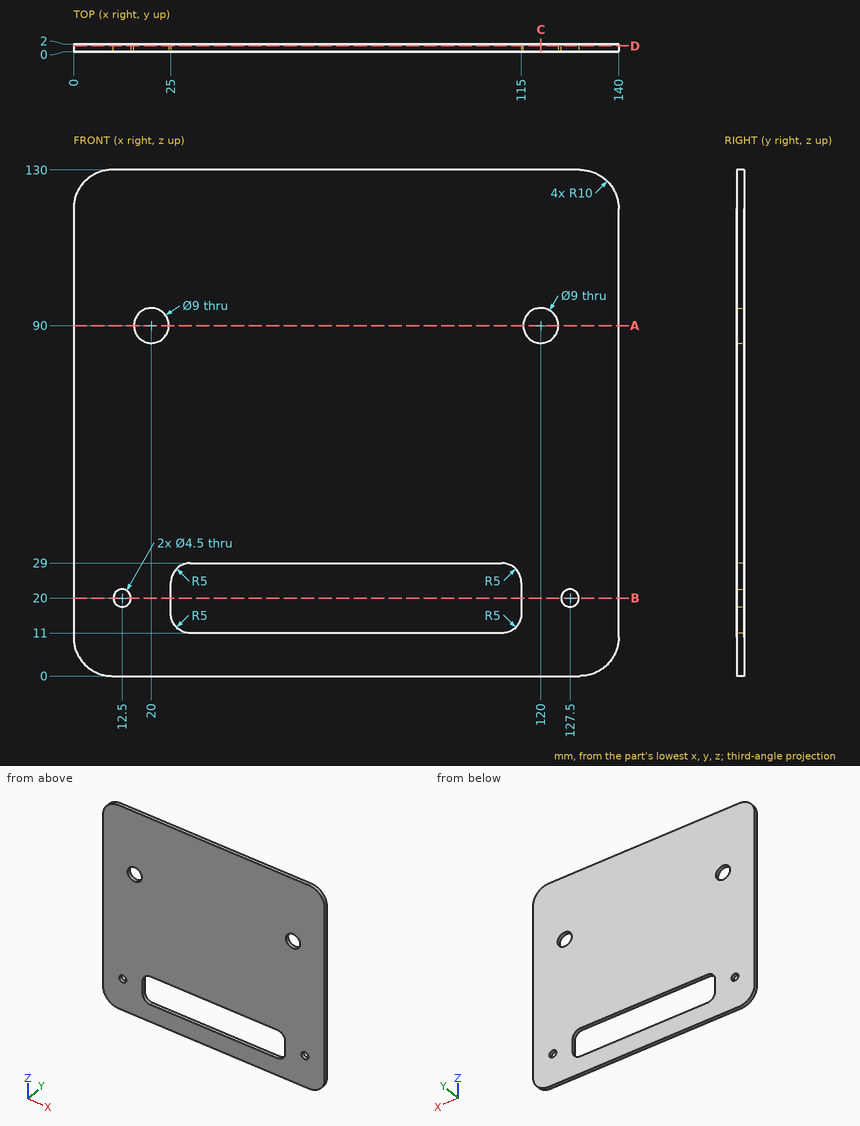
Geometry: see drawing. Coordinates: mm, zero at the bounding-box minimum. Coordinates: 2 decimals unless noted, no trailing zeros. Loops run counter-clockwise (first coordinate to the right, second up) from the corner with the lowest first, then second, coordinate; pieces in that order, holes last.
Q1. Contact query for a flat-ended pin moving along its axis: pin 1 (6 mm diameter, centred on x = 12.5, z = 20, fed in from -Y). Output: stop coordinate, or through.
Q2. Cut plane A-A (z = 90). Output: boundary loops of the cut face in (x, y), then the cut area to 3 significant figures.
Q3. Cut plane C-C (x = 120). Output: boundary loops of the cut face in (y, z), then the cut area to 3 significant figures.
Q4. Material intervals for line 1 (Z direction, x = 12.5, y = 1.4); line 2 (Z direction, x = 88, y = 0.6); line 3 (X direction, y = 0.4, z = 93.5), sorted ascending.
Q5. Cut plane B-B (z = 20). Output: boundary loops of the cut face in (x, y), then the cut area to 3 significant figures.
Q6. Cut plane D-D (y = 1.5). Output: boundary loops of the cut face in (x, z).
Working result:
1. pin 1: stops at y = 0
2. outline: (0, 0) - (15.5, 0) - (15.5, 2) - (0, 2) - close; (24.5, 0) - (115.5, 0) - (115.5, 2) - (24.5, 2) - close; (124.5, 0) - (140, 0) - (140, 2) - (124.5, 2) - close
2. area: 244 mm2
3. outline: (0, 0) - (2, 0) - (2, 85.5) - (0, 85.5) - close; (0, 94.5) - (2, 94.5) - (2, 130) - (0, 130) - close
3. area: 242 mm2
4. line 1: z = 0 to 17.75, 22.25 to 130
4. line 2: z = 0 to 11, 29 to 130
4. line 3: x = 0 to 17.17, 22.83 to 117.17, 122.83 to 140
5. outline: (0, 0) - (10.25, 0) - (10.25, 2) - (0, 2) - close; (14.75, 0) - (25, 0) - (25, 2) - (14.75, 2) - close; (115, 0) - (125.25, 0) - (125.25, 2) - (115, 2) - close; (129.75, 0) - (140, 0) - (140, 2) - (129.75, 2) - close
5. area: 82.0 mm2
6. outline: (0, 10) arc R10 ccw to (10, 0) - (130, 0) arc R10 ccw to (140, 10) - (140, 120) arc R10 ccw to (130, 130) - (10, 130) arc R10 ccw to (0, 120) - close; hole circle Ø4.5 at (12.5, 20); hole circle Ø9 at (20, 90); hole (25, 16) arc R5 ccw to (30, 11) - (110, 11) arc R5 ccw to (115, 16) - (115, 24) arc R5 ccw to (110, 29) - (30, 29) arc R5 ccw to (25, 24) - close; hole circle Ø9 at (120, 90); hole circle Ø4.5 at (127.5, 20)
